Autodesk Inventor part; units mm, degrees
ref_plane "Work Plane1" through (-33, -35, 0) normal (-1, 0, 0) x (0, 0, 1)
ref_plane "YZ Plane" through (0, 0, 0) normal (1, 0, 0) x (0, 1, 0)
ref_plane "XZ Plane" through (0, 0, 0) normal (0, 1, 0) x (-1, 0, 0)
sketch "Sketch1" plane through (0, 0, 0) normal (0, 0, 1) x (1, 0, 0)
  line L0 (85, -35) -> (55, -35)
  line L1 (55, -35) -> (55, 35)
  line L2 (55, 35) -> (85, 35)
  line L3 (85, 35) -> (85, -35)
  line L4 (85, -35) -> (55, 35) construction
  line L5 (55, -35) -> (85, 35) construction
  line L6 (-85, -35) -> (-55, -35)
  line L7 (-55, -35) -> (-55, 35)
  line L8 (-55, 35) -> (-85, 35)
  line L9 (-85, 35) -> (-85, -35)
  line L10 (-85, 35) -> (-85, 52.6783)
  line L11 (-85, -35) -> (-85, -52.6783)
  line L12 (85, 35) -> (85, 52.6783)
  line L13 (85, -35) -> (85, -52.6783)
  arc A0 (-85, -52.6783) -> (85, -52.6783) centre (0, 0) ccw
  arc A1 (85, 52.6783) -> (-85, 52.6783) centre (0, 0) ccw
  point P0 (70, 0)
  dimension "d6" = 30
  dimension "d7" = 70
  dimension "d155" = 100
extrude "Extrusion2" add sketch "Sketch1" along normal blind 3 contours L13 A0 L11 L6 L7 L8 L10 A1 L12 L2 L1 L0
sketch "Sketch3" plane through (0, 0, 0) normal (1, 0, 0) x (0, 1, 0)
  point P0 (0, 0)
ref_plane "Work Plane1" through (-33, -35, 0) normal (-1, 0, 0) x (0, 0, 1)
sketch "Sketch21" plane through (0, 0, 3) normal (0, 0, 1) x (1, 0, 0)
  line L0 (11, -59.3932) -> (11, -49.3932)
  line L1 (11, -49.3932) -> (-11, -49.3932)
  line L2 (-11, -49.3932) -> (11, -49.3932)
  line L3 (11, -49.3932) -> (11, -89.3932)
  line L4 (-11, -49.3932) -> (-11, -89.3932)
  line L5 (-11, -89.3932) -> (11, -89.3932)
  point P0 (0, 0)
  dimension "d149" = 40
sketch "Sketch31" plane through (0, 0, 3) normal (0, 0, 1) x (1, 0, 0)
  circle A0 centre (-56, -67.5) radius 1.5
  circle A1 centre (-56, -67.5) radius 1.5
  circle A2 centre (-25, -67.5) radius 1.5
  circle A3 centre (-25, -67.5) radius 1.5
  point P0 (0, 0)
  dimension "d117" = 3
  dimension "d118" = 3
extrude "Extrusion30" cut sketch "Sketch31" against normal up to next
mirror "Mirror19" about plane through (0, 0, 0) normal (0, 1, 0) of "Extrusion30"
mirror "Mirror20" about plane through (0, 0, 0) normal (1, 0, 0) of "Extrusion30", "Mirror19"
sketch "Sketch32" plane through (0, 0, 3) normal (0, 0, 1) x (1, 0, 0)
  line L0 (-33, 28) -> (-28, 28)
  line L1 (-28, 28) -> (-28, 20)
  line L2 (-33, 28) -> (-28, 28)
  line L3 (-28, 28) -> (-28, 20)
  line L4 (-28, 20) -> (-33, 20)
  line L5 (-33, 20) -> (-33, 28)
  line L6 (33, 28) -> (28, 28)
  line L7 (28, 28) -> (33, 28)
  line L8 (33, 28) -> (33, 20)
  line L9 (33, 20) -> (28, 20)
  line L10 (28, 20) -> (28, 28)
  point P0 (0, 0)
extrude "Extrusion31" cut sketch "Sketch32" against normal blind 1
sketch "Sketch33" plane through (0, 0, 0) normal (0, 0, -1) x (-1, 0, 0)
  line L0 (-60, 40) -> (-78, 40)
  line L1 (-78, 40) -> (-78, 46)
  line L2 (-78, 46) -> (-60, 46)
  line L3 (-60, 46) -> (-60, 40)
  point P0 (0, 0)
  dimension "d123" = 18
  dimension "d124" = 6
extrude "Extrusion32" cut sketch "Sketch33" against normal blind 1
mirror "Mirror21" about plane through (0, 0, 0) normal (1, 0, 0) of "Extrusion32"
mirror "Mirror22" about plane through (0, 0, 0) normal (0, 1, 0) of "Extrusion32", "Mirror21"
sketch "Sketch34" plane through (0, 0, 1) normal (0, 0, -1) x (-1, 0, 0)
  circle A0 centre (-75, 43) radius 1.5
  circle A1 centre (-63, 43) radius 1.5
  point P0 (0, 0)
  dimension "d127" = 3
  dimension "d128" = 3
extrude "Extrusion33" cut sketch "Sketch34" against normal up to next
mirror "Mirror23" about plane through (0, 0, 0) normal (1, 0, 0) of "Extrusion33"
mirror "Mirror24" about plane through (0, 0, 0) normal (0, 1, 0) of "Extrusion33", "Mirror23"
sketch "Sketch35" plane through (0, 0, 3) normal (0, 0, 1) x (1, 0, 0)
  point P0 (0, 0)
extrude "Extrusion35" cut sketch "Sketch21" against normal up to next
sketch "Sketch37" plane through (0, 0, 3) normal (0, 0, 1) x (1, 0, 0)
  line L0 (0, -58.4467) -> (16, -58.4467)
  circle A0 centre (16, -58.4467) radius 1.5
  circle A1 centre (16, -85) radius 1.5
  point P0 (0, 0)
  dimension "d137" = 16
  dimension "d138" = 3
  dimension "d139" = 3
extrude "Extrusion36" cut sketch "Sketch37" against normal up to next
mirror "Mirror25" about plane through (0, 0, 0) normal (1, 0, 0) of "Extrusion36"
sketch "Sketch38" plane through (0, 0, 3) normal (0, 0, 1) x (1, 0, 0)
  circle A0 centre (-25, -67.5) radius 1.5
  line L0 (-25, -67.5) -> (11, -67.5) construction
  circle A1 centre (-56, 67.5) radius 1.5
  circle A2 centre (-20, 67.5) radius 1.5
  circle A3 centre (-56, -67.5) radius 1.5
  line L1 (-56, -67.5) -> (-20, -67.5) construction
  circle A4 centre (-28.4224, -44.3596) radius 1.5
  point P0 (0, 0)
  dimension "d146" = 3
  dimension "d152" = 3
extrude "Extrusion38" cut sketch "Sketch38" against normal up to next contours A2 | A4
mirror "Mirror27" about plane through (0, 0, 0) normal (1, 0, 0) of "Extrusion38"
properties part number "底盤"
Input: part model. Units: mm. Frame: model coordinates. A direction names the side the tool comes from. Give positions to 0.01 mm unless a question says otherwise; leave off trailing zeros. Order: outer loops, then holes, each group sorted by start corner. A loop starts at its lowest first (then second) coordinate and runs counter-clockwise, first axis right, second up. Notation, with made-up numbers: (77, 46.25) - (86, 46.25) arc R14 ccw to (86, 65.25) - close; hole circle Ø2 at (17.5, -39). An arc over 180 degrees is marked (long way). Answer as a JSON object with one key per item and string values. Group by question number.
Q1. Line query: probe 1 along Y at (x, z) = (-71, 0.4); probe 2 along Y at (x, z) = (-16, 1); probe 3 along Y at (x, z) = (-2, 2.9). Output: solid intervals per line, ascending.
Q2. Cut plane A-A, the plane y = 23.5. Output: boundary loops of the cut face in (x, z).
Q3. First-contact query: pin 1 Ø1.1 at (x, z) = (68, 0.5) entering from -Y; pin 2 Ø3.5 at (x, y) = (16, -58.45) entering from +Z; pin 3 Ø1.8 at (x, y) = (-69, 42.5) entering from -Z; pin 4 Ø2.5 at (x, y) = (75, 43) entering from +Z. Flat tips, straight axial feed; report the tip coordinate or a pass-through.
Q4. Mould query, pull axis Y, two halves, no side actions, for faces 1 (the face through (-1.42, 99.99, 1.48)), 2 (the face through (-69, 43, 1)), 3 (the face through (30, 24, 2)), 4 (the face through (1.42, -99.99, 1.48)). Classes: pulls with the +Y half, pulls with the -Y half, needs draft (parallel to the pull), parting line crosses it, or undercut.
Q5. Set-up query: faces 5 (the face through (-1, 1, 0)), 6 (the face through (-31, 24, 2)), 7 (the face through (-69, -43, 1)). Return all of +Z, -Z, +X, -X, +Y, -Y with unobstructed straight access to the full face (end or side cutting, diameter ignored); none if empty.
Q6. Cut plane B-B, the plane z = 0.5. Count the separate pieces of the cut face and the enclosed holes in it, then the cut area to 3 significant figures.
Q7. Cut plane C-C, the plane x = 49. Output: boundary loops of the cut face in (y, z), then the cut area to 3 significant figures.
Q8. Cut plane D-D, the plane y = -4. Output: boundary loops of the cut face in (x, z).
Results:
{
 "1": {"probe 1": "-70.42 to -46, -40 to -35, 35 to 40, 46 to 70.42", "probe 2": "-98.71 to -86.5, -83.5 to -59.95, -56.95 to 98.71", "probe 3": "-99.98 to -89.39, -49.39 to 99.98"},
 "2": {"outline": "(-55, 0) - (55, 0) - (55, 3) - (33, 3) - (33, 2) - (28, 2) - (28, 3) - (-28, 3) - (-28, 2) - (-33, 2) - (-33, 3) - (-55, 3) - close"},
 "3": {"pin 1": "y = -73.83", "pin 2": "z = 3", "pin 3": "z = 1", "pin 4": "through"},
 "4": {"face 1": "pulls with the +Y half", "face 2": "undercut", "face 3": "undercut", "face 4": "pulls with the -Y half"},
 "5": {"face 5": "-Z, +X, -X, +Y, -Y", "face 6": "+Z", "face 7": "-Z"},
 "6": {"separate pieces": "1", "enclosed holes": "21", "area": "23,600 mm^2"},
 "7": {"outline": "(-87.17, 0) - (87.17, 0) - (87.17, 3) - (-87.17, 3) - close", "area": "523 mm^2"},
 "8": {"outline": "(-55, 0) - (55, 0) - (55, 3) - (-55, 3) - close"}
}
